Build history of the part. All positions in model axes, mm. Face numbers are marked on the shaded views. Coordinates: 2 decimals unless noted, no trailing zeros. Order: outer loops, then holes, each group sorted by start corner. A loop starts at its lowest first (then second) coordinate and runs counter-clockwise, first axis right, second up. Notation, with made-up numbers: (70.25, 6) - (74.25, 6) arc R24 ccw to (74.25, 33) - close; hole circle Ø6 at (61.5, 33). An arc over 180 degrees is marked (long way). Answer as CSV lines item,"result". Start each with the question number.
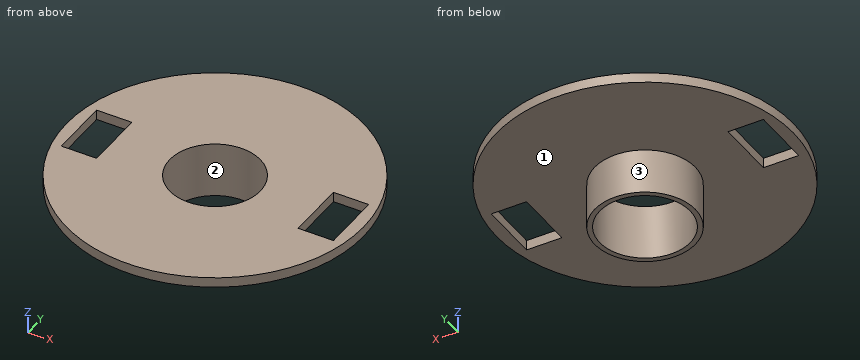
from build123d import *

# Parameters (mm, degrees)
SKETCH1_R           = 14.75
BOSS_EXTRUDE1_DEPTH = 1
SKETCH2_R           = 5
BOSS_EXTRUDE2_DEPTH = 4.5
SKETCH3_R           = 4.5
SKETCH3_W           = 3.5
SKETCH3_H           = 6
CUT_EXTRUDE1_DEPTH  = 6.5


with BuildPart() as part:
    # Sketch1 → Boss-Extrude1 (new body)
    with BuildSketch(Plane.XY):
        Circle(SKETCH1_R)
    extrude(amount=BOSS_EXTRUDE1_DEPTH)

    # Sketch2 → Boss-Extrude2 (add)
    with BuildSketch(Plane(origin=(0, 0, 0), x_dir=(-1, 0, 0), z_dir=(0, 0, -1))):
        Circle(SKETCH2_R)
    extrude(amount=BOSS_EXTRUDE2_DEPTH)

    # Sketch3 → Cut-Extrude1 (cut, through all)
    with BuildSketch(Plane(origin=(0, 0, -4.5), x_dir=(-1, 0, 0), z_dir=(0, 0, -1))):
        Circle(SKETCH3_R)
        with Locations((-11.75, 0)):
            Rectangle(SKETCH3_W, SKETCH3_H)
        with Locations((11.75, 0)):
            Rectangle(SKETCH3_W, SKETCH3_H)
    extrude(amount=-CUT_EXTRUDE1_DEPTH, mode=Mode.SUBTRACT)


solid = part.part
(1) Probe L1, parallel to Y at x = 0, z = -2.9; L2, parallel to X at y = -2.5, z = 0.4; L3, parallel to Z at x = 12.25, y = -5.25. List the from-to ranges inside material, lowest first. Write a range as [from, to].
(2) Band-saw the part on C-C on y = 0. List the corners of the cut face in (x, z), plus the area to 3 significant figures.
(3) Drop flat-ended pins along their axis: pin 1 Ø0.5 at (y, z) = (1.5, 0.5) entering from -X; pin 2 Ø0.5 at (y, z) = (-0.5, 0.5) entering from +X; pin 3 Ø0.5 at (x, z) = (-11.5, 0.5) entering from +Y. Give the stop position or say it passes through.
(4) Band-saw the part on B-B on x = 0. List the corners of the cut face in (y, z).
(5) Band-saw the part on A-A on z = 0.55. List the corners of the cut face in (x, y).
(6) Band-saw the part on D-D on z = -1.9. List the corners of the cut face in (x, y), plus the area to 3 significant figures.
(7) Pull direction Y, two halves, no side cores. Call the marked faces 1, 2 and 3: +Y half, -Y half, draft (parallel to the pull), parting line (faces both ways), or undercut.
Filled in:
1,L1,"y = [-5, -4.5], [4.5, 5]"
1,L2,"x = [-14.54, -13.5], [-10, -3.74], [3.74, 10], [13.5, 14.54]"
1,L3,"z = [0, 1]"
2,outline,"(-14.75, 0) - (-13.5, 0) - (-13.5, 1) - (-14.75, 1) - close; (-10, 0) - (-5, 0) - (-5, -4.5) - (-4.5, -4.5) - (-4.5, 1) - (-10, 1) - close; (4.5, -4.5) - (5, -4.5) - (5, 0) - (10, 0) - (10, 1) - (4.5, 1) - close; (13.5, 0) - (14.75, 0) - (14.75, 1) - (13.5, 1) - close"
2,area,"18.0 mm^2"
3,pin 1,"stops at x = -14.7"
3,pin 2,"stops at x = 14.75"
3,pin 3,"stops at y = 9.54"
4,outline,"(-14.75, 0) - (-5, 0) - (-5, -4.5) - (-4.5, -4.5) - (-4.5, 1) - (-14.75, 1) - close; (4.5, -4.5) - (5, -4.5) - (5, 0) - (14.75, 0) - (14.75, 1) - (4.5, 1) - close"
5,outline,"circle Ø29.5 at (0, 0); hole (-13.5, -3) - (-10, -3) - (-10, 3) - (-13.5, 3) - close; hole circle Ø9 at (0, 0); hole (10, -3) - (13.5, -3) - (13.5, 3) - (10, 3) - close"
6,outline,"circle Ø10 at (0, 0); hole circle Ø9 at (0, 0)"
6,area,"14.9 mm^2"
7,face 1,"draft"
7,face 2,"undercut"
7,face 3,"parting line"
